Check sheet for the drawn part. Datum: minimum x, y, z corner. Units: mm. A direction names the side the tool comes from. Coordinates: 2 decimals unless noted, no trailing zeros. Write each loop counter-clockwise with the first axis right and the second up, starting at its lowest first coordinate (ties: lowest second). Pieces come first, ordered by that corner, then holes. Notation, with made-up numbers: M 48.5,4 L 98.5,4 A16 cw 98.5,22 Z; hole C 47.25,-25 d2. An arc over 180 degrees is marked long. Answer as CSV lines item,"result".
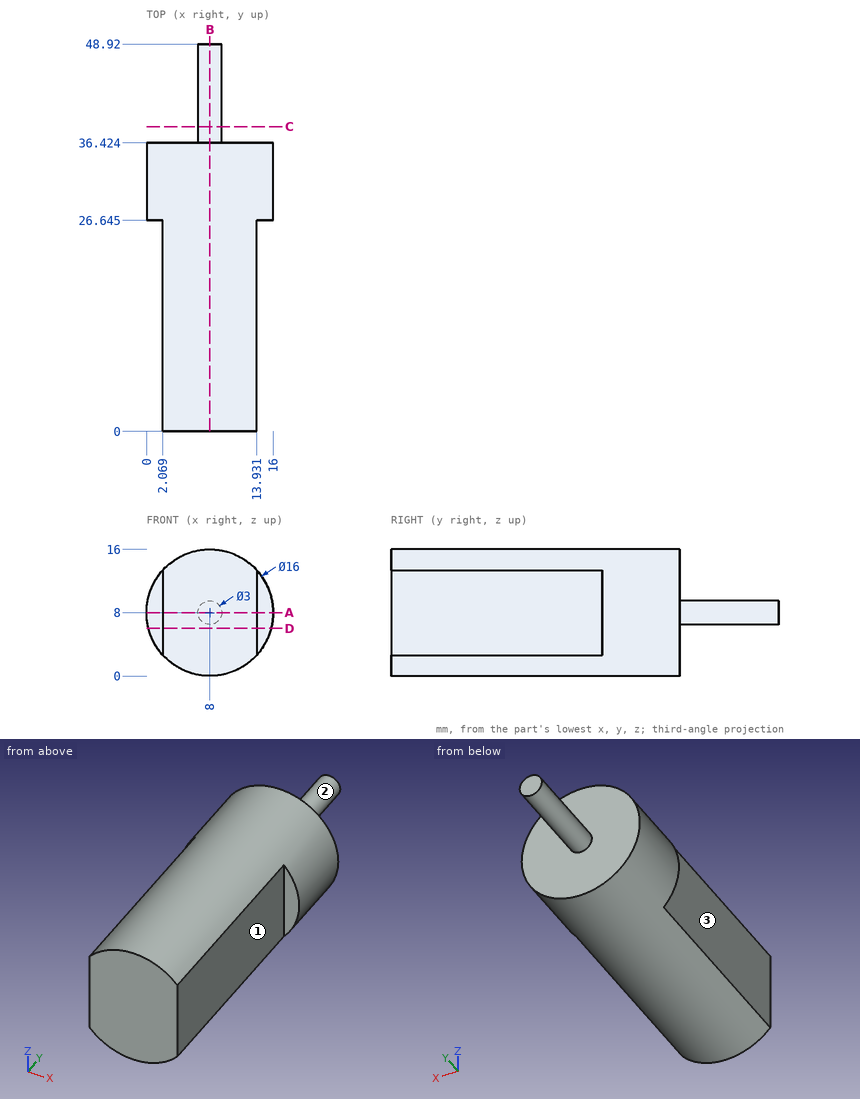
1) Section check C-C, the plane y = 38.5. Record the boundary of the cut face in (x, z).
Answer key:
outline,"C 8,8 d3"
2) Tool access check on the marked faces 1, 2 and 3. Record the directions out of +Z, -Z, +X, -X, +Y, -Y that give a thin tool (end or side, any length) a straight path to the whole face; none if there is none.
Answer key:
face 1,"+Z, -Z, +X, -Y"
face 2,"+Y"
face 3,"+Z, -Z, -X, -Y"
3) Section check D-D, the plane z = 6. Record the boundary of the cut face in (x, y) (1 decimal).
Answer key:
outline,"M 0.3,26.6 L 2.1,26.6 L 2.1,0 L 13.9,0 L 13.9,26.6 L 15.7,26.6 L 15.7,36.4 L 0.3,36.4 Z"
4) Depth check by flat-ended pin: P1, Ø1.5, axis at x = 3, y = 16.5, coming from the +Z side; P2, Ø2.5, axis at x = 1.5, z = 8, coming from the -Y side; P3, Ø6, axis at x = 3, y = 20, coming from the -Z side; P4, Ø1, axis at y = 16, z = 10, coming from the +X side. Enter the tip coordinate at first touch or a pass-through.
Answer key:
P1,"stops at z = 14.78"
P2,"stops at y = 0"
P3,"stops at z = 0.25"
P4,"stops at x = 13.93"
5) Section check A-A, the plane z = 8. Record the boundary of the cut face in (x, y) (1 decimal).
Answer key:
outline,"M 0,26.6 L 2.1,26.6 L 2.1,0 L 13.9,0 L 13.9,26.6 L 16,26.6 L 16,36.4 L 9.5,36.4 L 9.5,48.9 L 6.5,48.9 L 6.5,36.4 L 0,36.4 Z"
6) Thickness scan on line 1 along Y through (x, z) = (8.75, 4.5); line 2 along Y through (x, z) = (14.5, 5.75) (1 decimal); line 3 along X through (y, z) = (9, 8). Record the ranges inside material, lowest first.
Answer key:
line 1,"y = 0 to 36.42"
line 2,"y = 26.6 to 36.4"
line 3,"x = 2.07 to 13.93"
7) Section check B-B, the plane x = 8. Record the boundary of the cut face in (y, z), plus the area to 3 significant figures.
Answer key:
outline,"M 0,0 L 36.42,0 L 36.42,6.5 L 48.92,6.5 L 48.92,9.5 L 36.42,9.5 L 36.42,16 L 0,16 Z"
area,"620 mm2"
